```python
from build123d import *

# Parameters (mm, degrees)
F1_DEPTH = 21
F2_W     = 26
F2_H     = 17
F3_DEPTH = 25
F4_W     = 6
F4_H     = 7.4
F5_DEPTH = 25
F6_W     = 9
F6_H     = 4.6
F7_DEPTH = 1.5
F8_DEPTH = 3.5
F9_DEPTH = 3.001


with BuildPart() as f1:
    # F0 (on Front) → F1 (new body, symmetric)
    with BuildSketch(Plane.XZ):
        Polygon((-35, 0), (35, 0), (35, 3), (3.95, 3), (3.95, 10.4), (0, 10.4), (-3.95, 10.4), (-3.95, 3), (-35, 3), align=None)
    extrude(amount=F1_DEPTH, both=True)

    # F2 (on face) → F3 (cut)
    with BuildSketch(Plane(origin=(0, 0, 0), x_dir=(1, 0, 0), z_dir=(0, 0, -1))):
        with Locations((-22, 12.5)):
            Rectangle(F2_W, F2_H)
        with Locations((22, 12.5)):
            Rectangle(F2_W, F2_H)
    extrude(amount=-F3_DEPTH, mode=Mode.SUBTRACT)

    # F4 (on face) → F5 (cut)
    with BuildSketch(Plane(origin=(-3.95, 0, 0), x_dir=(0, -1, 0), z_dir=(-1, 0, 0))):
        with Locations((-18, 6.7)):
            Rectangle(F4_W, F4_H)
        with Locations((18, 6.7)):
            Rectangle(F4_W, F4_H)
    extrude(amount=-F5_DEPTH, mode=Mode.SUBTRACT)

    # F6 (on face) → F7 (join)
    with BuildSketch(Plane.XY.offset(3)):
        with Locations((-18, 14.7)):
            Rectangle(F6_W, F6_H)
        with Locations((-18, 3.3)):
            Rectangle(F6_W, F6_H)
        with Locations((18, 14.7)):
            Rectangle(F6_W, F6_H)
        with Locations((18, 3.3)):
            Rectangle(F6_W, F6_H)
    extrude(amount=F7_DEPTH)

    # F6 (on face) → F8 (join)
    with BuildSketch(Plane.XY.offset(3)):
        with BuildLine():
            Line((-13.5, 9.5), (-13.5, 11.4))
            Line((-13.5, 11.4), (-21, 11.4))
            Line((-21, 11.4), (-21, 9.5))
            Line((-21, 9.5), (-18.3956439237, 9.5))
            ThreePointArc((-18.3956439237, 9.5), (-17.25, 10.25), (-16.1043560763, 9.5))
            Line((-16.1043560763, 9.5), (-13.5, 9.5))
        make_face()
        with BuildLine():
            Line((-13.5, 6.6), (-13.5, 8.5))
            Line((-13.5, 8.5), (-16.1043560763, 8.5))
            ThreePointArc((-16.1043560763, 8.5), (-17.25, 7.75), (-18.3956439237, 8.5))
            Line((-18.3956439237, 8.5), (-21, 8.5))
            Line((-21, 8.5), (-21, 6.6))
            Line((-21, 6.6), (-13.5, 6.6))
        make_face()
        with BuildLine():
            Line((21, 11.4), (13.5, 11.4))
            Line((13.5, 11.4), (13.5, 9.5))
            Line((13.5, 9.5), (16.1043560763, 9.5))
            ThreePointArc((16.1043560763, 9.5), (17.25, 10.25), (18.3956439237, 9.5))
            Line((18.3956439237, 9.5), (21, 9.5))
            Line((21, 9.5), (21, 11.4))
        make_face()
        with BuildLine():
            Line((13.5, 8.5), (13.5, 6.6))
            Line((13.5, 6.6), (21, 6.6))
            Line((21, 6.6), (21, 8.5))
            Line((21, 8.5), (18.3956439237, 8.5))
            ThreePointArc((18.3956439237, 8.5), (17.25, 7.75), (16.1043560763, 8.5))
            Line((16.1043560763, 8.5), (13.5, 8.5))
        make_face()
    extrude(amount=F8_DEPTH)

    # F6 (on face) → F9 (cut, through all)
    with BuildSketch(Plane.XY.offset(3)):
        with BuildLine():
            Line((-13.5, 8.5), (-13.5, 9.5))
            Line((-13.5, 9.5), (-16.1043560763, 9.5))
            ThreePointArc((-16.1043560763, 9.5), (-16.0263671088, 9.2553870546), (-16, 9))
            ThreePointArc((-16, 9), (-16.0263671088, 8.7446129454), (-16.1043560763, 8.5))
            Line((-16.1043560763, 8.5), (-13.5, 8.5))
        make_face()
        with BuildLine():
            ThreePointArc((-16, 9), (-16.0263671088, 9.2553870546), (-16.1043560763, 9.5))
            Line((-16.1043560763, 9.5), (-18.3956439237, 9.5))
            ThreePointArc((-18.3956439237, 9.5), (-18.5, 9), (-18.3956439237, 8.5))
            Line((-18.3956439237, 8.5), (-16.1043560763, 8.5))
            ThreePointArc((-16.1043560763, 8.5), (-16.0263671088, 8.7446129454), (-16, 9))
        make_face()
        with BuildLine():
            Line((-18.3956439237, 9.5), (-21, 9.5))
            Line((-21, 9.5), (-21, 8.5))
            Line((-21, 8.5), (-18.3956439237, 8.5))
            ThreePointArc((-18.3956439237, 8.5), (-18.5, 9), (-18.3956439237, 9.5))
        make_face()
        with BuildLine():
            Line((16.1043560763, 9.5), (13.5, 9.5))
            Line((13.5, 9.5), (13.5, 8.5))
            Line((13.5, 8.5), (16.1043560763, 8.5))
            ThreePointArc((16.1043560763, 8.5), (16, 9), (16.1043560763, 9.5))
        make_face()
        with BuildLine():
            Line((18.3956439237, 9.5), (16.1043560763, 9.5))
            ThreePointArc((16.1043560763, 9.5), (16, 9), (16.1043560763, 8.5))
            Line((16.1043560763, 8.5), (18.3956439237, 8.5))
            ThreePointArc((18.3956439237, 8.5), (18.4736328912, 8.7446129454), (18.5, 9))
            ThreePointArc((18.5, 9), (18.4736328912, 9.2553870546), (18.3956439237, 9.5))
        make_face()
        with BuildLine():
            Line((21, 8.5), (21, 9.5))
            Line((21, 9.5), (18.3956439237, 9.5))
            ThreePointArc((18.3956439237, 9.5), (18.4736328912, 9.2553870546), (18.5, 9))
            ThreePointArc((18.5, 9), (18.4736328912, 8.7446129454), (18.3956439237, 8.5))
            Line((18.3956439237, 8.5), (21, 8.5))
        make_face()
        with BuildLine():
            Line((-18.3956439237, 9.5), (-16.1043560763, 9.5))
            ThreePointArc((-16.1043560763, 9.5), (-17.25, 10.25), (-18.3956439237, 9.5))
        make_face()
        with BuildLine():
            ThreePointArc((-18.3956439237, 8.5), (-17.25, 7.75), (-16.1043560763, 8.5))
            Line((-16.1043560763, 8.5), (-18.3956439237, 8.5))
        make_face()
        with BuildLine():
            ThreePointArc((18.3956439237, 9.5), (17.25, 10.25), (16.1043560763, 9.5))
            Line((16.1043560763, 9.5), (18.3956439237, 9.5))
        make_face()
        with BuildLine():
            Line((18.3956439237, 8.5), (16.1043560763, 8.5))
            ThreePointArc((16.1043560763, 8.5), (17.25, 7.75), (18.3956439237, 8.5))
        make_face()
    extrude(amount=-F9_DEPTH, mode=Mode.SUBTRACT)


solid = f1.part
```
CAD build for the part. Positions are in the model's coordinates, mm. A direction names the side the tool comes from. Coordinates: 2 decimals unless noted, no trailing zeros. Order: outer loops, then holes, each group sorted by start corner. A loop starts at its lowest first (then second) coordinate and runs counter-clockwise, first axis right, second up. Notation, with made-up numbers: M 18,60.25 L 49,60.25 A18 cw 49,76.25 Z; hole C -12.5,59 d10. An arc over 180 degrees is marked long. Write each question's results on one line, items separated by ' | '. Start each with the question number.
Q1. Cut at D-D (z = 7.25). List the corners of the cut face in (x, y).
Q2. Pull direction Y, two halves, no side cores. Call faces 4 (the flat face through (18, 5.6, 4)), 5 (the flat face through (0, -21, 2)), 6 (the flat face through (13.5, 15, 4)): +Y half, -Y half, draft (parallel to the pull), parting line (faces both ways), or undercut.
Q3. Cut at A-A (z = 2). List the corners of the cut face in (x, y), then the cut area to 3 significant figures.
Q4. Cut at B-B (y = -10). List the corners of the cut face in (x, z).
Q5. Flat gauge pins, fed straight in: P1, Ø1.5, axis at x = -23, z = 4.5, coming from the -Y side; P2, Ø3, axis at x = -17.5, z = 4, coming from the -Y side; P3, Ø1, axis at x = -4.5, y = 0, coming from the +Z side. Where does each tip first touch, or does it go through?
Q6. Cut at C-C (x = 5.5). List the corners of the cut face in (y, z).
Q7. Drill centre lines: probe 1 along Z at (x, y) = (7, -0.5); probe 2 along X at (y, z) = (-7, 3.75); probe 3 along X at (y, z) = (-4.5, 2.25). Where is each one in solid material? Low to high. Write a range as from..to.
Q8. Which spindle directions (+Z, -Z, +X, -X, +Y, -Y) get a long thin tool onto all of the face, cutting with end or side? Do faces 1 (the flat face through (13.5, 8, 5)), 2 (the flat face through (21, 10, 5)), 3 (the flat face through (-20, 9.5, 3)). Say none if no direction does.
Found:
1) outline: M -3.95,-15 L 3.95,-15 L 3.95,15 L -3.95,15 Z
2) face 4: undercut | face 5: -Y half | face 6: draft
3) outline: M -35,-4 L -9,-4 L -9,-21 L 9,-21 L 9,-4 L 35,-4 L 35,21 L -35,21 Z; hole M -21,8.5 L -18.4,8.5 A1.25 ccw -16.1,8.5 L -13.5,8.5 L -13.5,9.5 L -16.1,9.5 A1.25 ccw -18.4,9.5 L -21,9.5 Z; hole M 13.5,8.5 L 16.1,8.5 A1.25 ccw 18.4,8.5 L 21,8.5 L 21,9.5 L 18.4,9.5 A1.25 ccw 16.1,9.5 L 13.5,9.5 Z | area: 2,040 mm²
4) outline: M -9,0 L 9,0 L 9,3 L 3.95,3 L 3.95,10.4 L -3.95,10.4 L -3.95,3 L -9,3 Z
5) P1: y = 1 | P2: y = -4 | P3: z = 3
6) outline: M -21,0 L 21,0 L 21,3 L -21,3 Z
7) probe 1: 0..3 | probe 2: -3.95..3.95 | probe 3: -9..9
8) face 1: +Z, +Y, -Y | face 2: +Z, +X | face 3: +Z, -Z
